from build123d import *

# Parameters (mm, degrees)
SKETCH1_W                = 10
SKETCH1_H                = 14.198074023
BOSS_EXTRUDE1_DEPTH      = 337.560694
BOSS_EXTRUDE1_2_DEPTH    = 337.560694
BOSS_EXTRUDE1_3_DEPTH    = 337.560694
BOSS_EXTRUDE1_4_DEPTH    = 337.560694
BOSS_EXTRUDE1_5_DEPTH    = 337.560694
BOSS_EXTRUDE1_6_DEPTH    = 337.560694
BOSS_EXTRUDE1_7_DEPTH    = 337.560694
BOSS_EXTRUDE1_8_DEPTH    = 337.560694
BOSS_EXTRUDE1_9_DEPTH    = 337.560694
BOSS_EXTRUDE1_10_DEPTH   = 337.560694
BOSS_EXTRUDE1_11_DEPTH   = 337.560694
BOSS_EXTRUDE1_12_DEPTH   = 337.560694
BOSS_EXTRUDE1_13_DEPTH   = 337.560694
BOSS_EXTRUDE1_14_DEPTH   = 337.560694
BOSS_EXTRUDE1_15_DEPTH   = 337.560694
SKETCH2_W                = 290
SKETCH2_H                = 4.038074023
BOSS_EXTRUDE2_DEPTH      = 10
BOSS_EXTRUDE2_DEPTH_BACK = 10
SKETCH3_W                = 290
SKETCH3_H                = 4.038074023
BOSS_EXTRUDE3_DEPTH      = 10
BOSS_EXTRUDE3_DEPTH_BACK = 10
SKETCH4_W                = 357.560693512
SKETCH4_H                = 4.038074023
BOSS_EXTRUDE4_DEPTH      = 12
BOSS_EXTRUDE6_DEPTH      = 17


with BuildPart() as part:
    # Sketch1 → Boss-Extrude1 (new body)
    with BuildSketch(Plane.XY):
        with Locations((-5.671527203, 329.103441202)):
            Rectangle(SKETCH1_W, SKETCH1_H)
    extrude(amount=BOSS_EXTRUDE1_DEPTH)



with BuildPart() as body_2:
    # Sketch1 → Boss-Extrude1 2 (new body)
    with BuildSketch(Plane.XY):
        with Locations((-25.671527203, 329.103441202)):
            Rectangle(SKETCH1_W, SKETCH1_H)
    extrude(amount=BOSS_EXTRUDE1_2_DEPTH)


with BuildPart() as body_3:
    # Sketch1 → Boss-Extrude1 3 (new body)
    with BuildSketch(Plane.XY):
        with Locations((-45.671527203, 329.103441202)):
            Rectangle(SKETCH1_W, SKETCH1_H)
    extrude(amount=BOSS_EXTRUDE1_3_DEPTH)


with BuildPart() as body_4:
    # Sketch1 → Boss-Extrude1 4 (new body)
    with BuildSketch(Plane.XY):
        with Locations((-65.671527203, 329.103441202)):
            Rectangle(SKETCH1_W, SKETCH1_H)
    extrude(amount=BOSS_EXTRUDE1_4_DEPTH)


with BuildPart() as body_5:
    # Sketch1 → Boss-Extrude1 5 (new body)
    with BuildSketch(Plane.XY):
        with Locations((-85.671527203, 329.103441202)):
            Rectangle(SKETCH1_W, SKETCH1_H)
    extrude(amount=BOSS_EXTRUDE1_5_DEPTH)


with BuildPart() as body_6:
    # Sketch1 → Boss-Extrude1 6 (new body)
    with BuildSketch(Plane.XY):
        with Locations((-105.671527203, 329.103441202)):
            Rectangle(SKETCH1_W, SKETCH1_H)
    extrude(amount=BOSS_EXTRUDE1_6_DEPTH)


with BuildPart() as body_7:
    # Sketch1 → Boss-Extrude1 7 (new body)
    with BuildSketch(Plane.XY):
        with Locations((-125.671527203, 329.103441202)):
            Rectangle(SKETCH1_W, SKETCH1_H)
    extrude(amount=BOSS_EXTRUDE1_7_DEPTH)


with BuildPart() as body_8:
    # Sketch1 → Boss-Extrude1 8 (new body)
    with BuildSketch(Plane.XY):
        with Locations((-145.671527203, 329.103441202)):
            Rectangle(SKETCH1_W, SKETCH1_H)
    extrude(amount=BOSS_EXTRUDE1_8_DEPTH)


with BuildPart() as body_9:
    # Sketch1 → Boss-Extrude1 9 (new body)
    with BuildSketch(Plane.XY):
        with Locations((-165.671527203, 329.103441202)):
            Rectangle(SKETCH1_W, SKETCH1_H)
    extrude(amount=BOSS_EXTRUDE1_9_DEPTH)


with BuildPart() as body_10:
    # Sketch1 → Boss-Extrude1 10 (new body)
    with BuildSketch(Plane.XY):
        with Locations((-185.671527203, 329.103441202)):
            Rectangle(SKETCH1_W, SKETCH1_H)
    extrude(amount=BOSS_EXTRUDE1_10_DEPTH)


with BuildPart() as body_11:
    # Sketch1 → Boss-Extrude1 11 (new body)
    with BuildSketch(Plane.XY):
        with Locations((-205.671527203, 329.103441202)):
            Rectangle(SKETCH1_W, SKETCH1_H)
    extrude(amount=BOSS_EXTRUDE1_11_DEPTH)


with BuildPart() as body_12:
    # Sketch1 → Boss-Extrude1 12 (new body)
    with BuildSketch(Plane.XY):
        with Locations((-225.671527203, 329.103441202)):
            Rectangle(SKETCH1_W, SKETCH1_H)
    extrude(amount=BOSS_EXTRUDE1_12_DEPTH)


with BuildPart() as body_13:
    # Sketch1 → Boss-Extrude1 13 (new body)
    with BuildSketch(Plane.XY):
        with Locations((-245.671527203, 329.103441202)):
            Rectangle(SKETCH1_W, SKETCH1_H)
    extrude(amount=BOSS_EXTRUDE1_13_DEPTH)


with BuildPart() as body_14:
    # Sketch1 → Boss-Extrude1 14 (new body)
    with BuildSketch(Plane.XY):
        with Locations((-265.671527203, 329.103441202)):
            Rectangle(SKETCH1_W, SKETCH1_H)
    extrude(amount=BOSS_EXTRUDE1_14_DEPTH)


with BuildPart() as body_15:
    # Sketch1 → Boss-Extrude1 15 (new body)
    with BuildSketch(Plane.XY):
        with Locations((-285.671527203, 329.103441202)):
            Rectangle(SKETCH1_W, SKETCH1_H)
    extrude(amount=BOSS_EXTRUDE1_15_DEPTH)


with BuildPart() as part_1:
    add(part.part)

    add(body_2.part)  # Boss-Extrude2 merges body 2

    add(body_3.part)  # Boss-Extrude2 merges body 3

    add(body_4.part)  # Boss-Extrude2 merges body 4

    add(body_5.part)  # Boss-Extrude2 merges body 5

    add(body_6.part)  # Boss-Extrude2 merges body 6

    add(body_7.part)  # Boss-Extrude2 merges body 7

    add(body_8.part)  # Boss-Extrude2 merges body 8

    add(body_9.part)  # Boss-Extrude2 merges body 9

    add(body_10.part)  # Boss-Extrude2 merges body 10

    add(body_11.part)  # Boss-Extrude2 merges body 11

    add(body_12.part)  # Boss-Extrude2 merges body 12

    add(body_13.part)  # Boss-Extrude2 merges body 13

    add(body_14.part)  # Boss-Extrude2 merges body 14

    add(body_15.part)  # Boss-Extrude2 merges body 15
    # Sketch2 → Boss-Extrude2 (add, two sides)
    with BuildSketch(Plane.XY.offset(337.560693512)) as boss_extrude2_sk:
        with Locations((-145.671527203, 324.023441203)):
            Rectangle(SKETCH2_W, SKETCH2_H)
    extrude(amount=BOSS_EXTRUDE2_DEPTH)
    extrude(boss_extrude2_sk.sketch, amount=-BOSS_EXTRUDE2_DEPTH_BACK)

    # Sketch3 → Boss-Extrude3 (add, two sides)
    with BuildSketch(Plane(origin=(0, 0, 0), x_dir=(-1, 0, 0), z_dir=(0, 0, -1))) as boss_extrude3_sk:
        with Locations((145.671527203, 324.023441203)):
            Rectangle(SKETCH3_W, SKETCH3_H)
    extrude(amount=BOSS_EXTRUDE3_DEPTH)
    extrude(boss_extrude3_sk.sketch, amount=-BOSS_EXTRUDE3_DEPTH_BACK)

    # Sketch4 → Boss-Extrude4 (add)
    with BuildSketch(Plane(origin=(-0.671527203, 0, 0), x_dir=(0, 0, -1), z_dir=(1, 0, 0))):
        with Locations((-168.780346756, 324.023441203)):
            Rectangle(SKETCH4_W, SKETCH4_H)
    extrude(amount=BOSS_EXTRUDE4_DEPTH)

    # Sketch5 → Boss-Extrude6 (add)
    with BuildSketch(Plane.ZY.offset(290.671527203)):
        Polygon((337.560693512, 326.042478214), (0, 326.042478214), (-10, 326.042478214), (-10, 322.004404191), (347.560693512, 322.004404191), (347.560693512, 326.042478214), align=None)
    extrude(amount=BOSS_EXTRUDE6_DEPTH)


solid = part_1.part
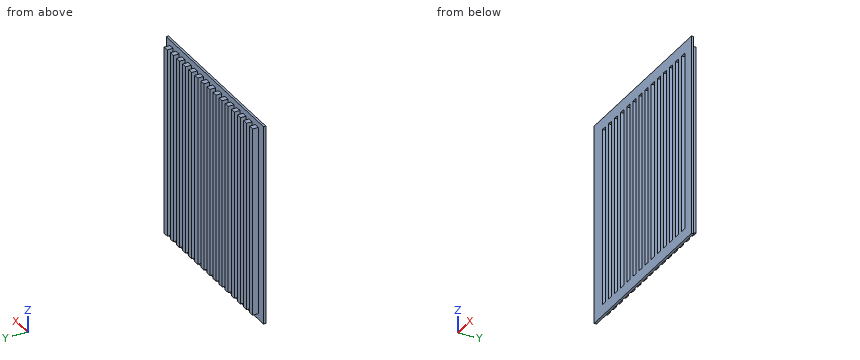
Model file for the job. Use its own axes, mm. Round coordinates to 2 decimals unless told otherwise and drop trailing zeros. Loops run counter-clockwise (first coordinate to the right, second up) from the corner with the lowest first, then second, coordinate; pieces in that order, holes last. Notation, with made-up numbers: M -29.5,-20.75 L -3.5,-20.75 A19 cw -3.5,14.25 Z; hole C 87,41 d9. An arc over 180 degrees is marked long. One line per question, with ' | ' between items.
1) Flat gauge pins, fed straight in: pin 1 (3 mm diameter, centred on x = -266, y = 329.5, fed in from -Z); pin 2 (4.5 mm diameter, centred on y = 329, z = 134, fed in from -X); pin 3 (5 mm diameter, centred on x = -93, y = 333.5, fed in from +Z). Where does each tip first touch, or does it go through?
Solved:
pin 1: stops at z = 0 | pin 2: stops at x = -290.67 | pin 3: stops at z = 337.56
2) Band-saw the part on B-B (x = -226). Give the cut face in (y, z).
Solved:
outline: M 322,-10 L 326.04,-10 L 326.04,0 L 336.2,0 L 336.2,337.56 L 326.04,337.56 L 326.04,347.56 L 322,347.56 Z
3) Drill centre lines: line 1 along Z through (x, y) = (-120, 325.25); line 2 along Z through (x, y) = (-246, 332.25). Where is each one in solid material? Low to high.
Solved:
line 1: z = -10 to 10, 327.56 to 347.56 | line 2: z = 0 to 337.56
4) Band-saw the part on A-A (x = -136). Give the cut face in (y, z), then the cut area to 3 significant figures.
Solved:
outline: M 322,-10 L 326.04,-10 L 326.04,10 L 322,10 Z; M 322,327.56 L 326.04,327.56 L 326.04,347.56 L 322,347.56 Z | area: 162 mm²
5) Band-saw the part on C-C (z = 260). Give the number of separate pieces and of enclosed holes in the cut face, then the cut area to 3 significant figures.
Solved:
separate pieces: 15 | enclosed holes: 0 | area: 2,250 mm²
